The model under review builds one solid part; all positions refer to its coordinate system, in mm. Give positions to 0.01 mm unless a question says otherwise; leave off trailing zeros. Order: outer loops, then holes, each group sorted by start corner. A loop starts at its lowest first (then second) coordinate and runs counter-clockwise, first axis right, second up. Notation, with made-up numbers: (-24, 3) -> (-15, 3) arc R30 ccw to (-15, 26) -> close; hole circle Ø9 at (53, 83). An arc over 180 degrees is marked (long way). Use one line per item in the form item = value.
```python
from build123d import *

# Parameters (mm, degrees)
ESQUISSE1_W                                    = 275
ESQUISSE1_H                                    = 205
BOSS_EXTRU_1_DEPTH                             = 5
FRAISAGE_POUR_VIS_T_TE_FRAIS_E_M41_D           = 4.8
FRAISAGE_POUR_VIS_T_TE_FRAIS_E_M41_CSINK_D     = 9.4
FRAISAGE_POUR_VIS_T_TE_FRAIS_E_M41_CSINK_ANGLE = 90
ESQUISSE5_W                                    = 10
ESQUISSE5_H                                    = 10
ENL_V_MAT_EXTRU_1_DEPTH                        = 1
ENL_V_MAT_EXTRU_2_DEPTH                        = 172.573599368
ENL_V_MAT_EXTRU_2_DEPTH_BACK                   = 172.573599368
ESQUISSE9_R                                    = 22.5
D_GAGEMENT_M32_D                               = 3.4
D_GAGEMENT_M32_DEPTH                           = 12
D_GAGEMENT_M32_TIP                             = 1.021463052
ESQUISSE16_W                                   = 100
ESQUISSE16_H                                   = 5
BOSS_EXTRU_2_DEPTH                             = 7
ESQUISSE18_W                                   = 100
ESQUISSE18_H                                   = 2.5
ENL_V_MAT_EXTRU_3_DEPTH                        = 1.7
ESQUISSE17_W                                   = 100
ESQUISSE17_H                                   = 2.5
ENL_V_MAT_EXTRU_4_DEPTH                        = 1.7
BOSS_EXTRU_4_DEPTH                             = 7
ESQUISSE21_W                                   = 20.5
ESQUISSE21_H                                   = 6.5
ENL_V_MAT_EXTRU_5_DEPTH                        = 13


with BuildPart() as part:
    # Esquisse1 → Boss.-Extru.1 (new body)
    with BuildSketch(Plane(origin=(0, 0, 0), x_dir=(1, 0, 0), z_dir=(0, 1, 0))):
        Rectangle(ESQUISSE1_W, ESQUISSE1_H)
    extrude(amount=BOSS_EXTRU_1_DEPTH)

    # Fraisage pour vis à tête fraisée M41 (through all)
    with Locations(Plane(origin=(0, 5, 0), x_dir=(1, 0, 0), z_dir=(0, 1, 0))):
        with Locations((-131.5, 96.5), (-131.5, -96.5), (131.5, -96.5), (131.5, 96.5)):
            CounterSinkHole(FRAISAGE_POUR_VIS_T_TE_FRAIS_E_M41_D / 2, FRAISAGE_POUR_VIS_T_TE_FRAIS_E_M41_CSINK_D / 2, counter_sink_angle=FRAISAGE_POUR_VIS_T_TE_FRAIS_E_M41_CSINK_ANGLE)

    # Esquisse5 → Enlèv. mat.-Extru.1 (cut)
    with BuildSketch(Plane(origin=(0, 5, 0), x_dir=(1, 0, 0), z_dir=(0, 1, 0))):
        with Locations((-87.5, 79)):
            Rectangle(ESQUISSE5_W, ESQUISSE5_H)
        with Locations((117.5, 79)):
            Rectangle(ESQUISSE5_W, ESQUISSE5_H)
        with Locations((117.5, -79)):
            Rectangle(ESQUISSE5_W, ESQUISSE5_H)
        with Locations((-87.5, -79)):
            Rectangle(ESQUISSE5_W, ESQUISSE5_H)
    extrude(amount=-ENL_V_MAT_EXTRU_1_DEPTH, mode=Mode.SUBTRACT)

    # Esquisse9 → Enlèv. mat.-Extru.2 (cut, two sides: drawn at the far end of the back side and taken through both)
    with BuildSketch(Plane(origin=(0, 5, 0), x_dir=(1, 0, 0), z_dir=(0, 1, 0)).offset(-ENL_V_MAT_EXTRU_2_DEPTH_BACK)):
        with Locations(Location((13, 0, 0), (0, 0, 270))):
            Circle(ESQUISSE9_R)
    extrude(amount=ENL_V_MAT_EXTRU_2_DEPTH + ENL_V_MAT_EXTRU_2_DEPTH_BACK, mode=Mode.SUBTRACT)

    # Dégagement M32
    with Locations(Plane(origin=(0, 4, 0), x_dir=(1, 0, 0), z_dir=(0, 1, 0))):
        with Locations((-87.5, -79), (-87.5, 79), (117.5, 79), (117.5, -79)):
            Hole(D_GAGEMENT_M32_D / 2, depth=D_GAGEMENT_M32_DEPTH)
            with Locations((0, 0, -(D_GAGEMENT_M32_DEPTH + D_GAGEMENT_M32_TIP / 2))):  # 118° drill point
                Cone(0, D_GAGEMENT_M32_D / 2, D_GAGEMENT_M32_TIP, mode=Mode.SUBTRACT)

    # Esquisse16 → Boss.-Extru.2 (add)
    with BuildSketch(Plane.XZ):
        with Locations((-15, 30.5)):
            Rectangle(ESQUISSE16_W, ESQUISSE16_H)
        with Locations((-15, -30.5)):
            Rectangle(ESQUISSE16_W, ESQUISSE16_H)
    extrude(amount=BOSS_EXTRU_2_DEPTH)

    # Esquisse18 → Enlèv. mat.-Extru.3 (cut)
    with BuildSketch(Plane(origin=(0, 0, 28), x_dir=(-1, 0, 0), z_dir=(0, 0, -1))):
        with Locations((15, -1.25)):
            Rectangle(ESQUISSE18_W, ESQUISSE18_H)
    extrude(amount=-ENL_V_MAT_EXTRU_3_DEPTH, mode=Mode.SUBTRACT)

    # Esquisse17 → Enlèv. mat.-Extru.4 (cut)
    with BuildSketch(Plane.XY.offset(-28)):
        with Locations((-15, -1.25)):
            Rectangle(ESQUISSE17_W, ESQUISSE17_H)
    extrude(amount=-ENL_V_MAT_EXTRU_4_DEPTH, mode=Mode.SUBTRACT)

    # Esquisse19 → Boss.-Extru.4 (add)
    with BuildSketch(Plane(origin=(0, 0, 0), x_dir=(-1, 0, 0), z_dir=(0, -1, 0))):
        Polygon((-35, -33), (-40, -33), (-45, -33), (-45, -3.794590368), (-40, -3.794590368), (-40, 33), (-35, 33), (-35, 3.79695048), (-35.5, 0), (-35, -3.794590368), align=None)
    extrude(amount=BOSS_EXTRU_4_DEPTH)

    # Esquisse21 → Enlèv. mat.-Extru.5 (cut)
    with BuildSketch(Plane.ZY.offset(-35)):
        with Locations((15.149590368, -3.5)):
            Rectangle(ESQUISSE21_W, ESQUISSE21_H)
    extrude(amount=-ENL_V_MAT_EXTRU_5_DEPTH, mode=Mode.SUBTRACT)


solid = part.part
```
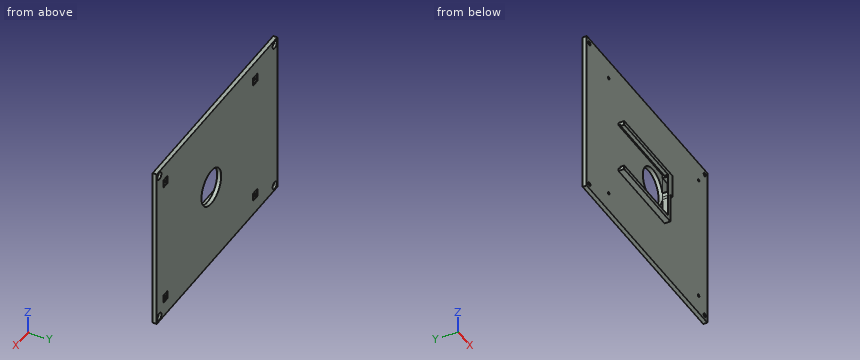
1. For pin 1 Ø5.5 at (x, y) = (42.5, -4.5) entering from -Z; pin 2 Ø0.8 at (x, y) = (-13, -1.5) entering from +Z; pin 3 Ø8 at (x, z) = (-58, -22) entering from -Y, all flat-tipped, find the tip position at first contact; note any pin that passes through.
Values:
pin_1 = -33
pin_2 = 33
pin_3 = 0
2. Add section A-A on x = -48. Give the boundary of the cut face in (y, z).
Values:
outline = (-7, -33) -> (0, -33) -> (0, -102.5) -> (5, -102.5) -> (5, 102.5) -> (0, 102.5) -> (0, 33) -> (-7, 33) -> (-7, 28) -> (-2.5, 28) -> (-2.5, 29.7) -> (0, 29.7) -> (0, -29.7) -> (-2.5, -29.7) -> (-2.5, -28) -> (-7, -28) -> close
3. Add section B-B on z = 45.5. Give the boundary of the cut face in (x, y).
Values:
outline = (-137.5, 0) -> (137.5, 0) -> (137.5, 5) -> (-137.5, 5) -> close
4. For L1, parallel to Z at x = 117.5, y = 2.4; L2, parallel to Z at x = 131.5, y = 1.9; L3, parallel to X at y = 2.6, z = 79, list the stretches that pass through material, from the lowest coordinate up.
Values:
L1 = -102.5 to -80.7, -77.3 to 77.3, 80.7 to 102.5
L2 = -102.5 to -98.9, -94.1 to 94.1, 98.9 to 102.5
L3 = -137.5 to -89.2, -85.8 to 115.8, 119.2 to 137.5
